For this review, take the finished solid that the model builds, in its own axes (mm). Face numbers are marked on the shaded views. A direction names the side the tool comes from. Coordinates: 2 decimals unless noted, no trailing zeros. Write each loop counter-clockwise with the first axis right and the second up, starting at its lowest first coordinate (ties: lowest second). Pieces come first, ordered by that corner, then holes.
1) We need section B-B on x = 80. Write out the cut boundary in (y, z), then the cut area to 3 significant figures.
2) Mouldability with a two-part tool opening along X and no side actions: class the marked faces 1 and 2 as pulls with the +X half, pulls with the -X half, needs draft (parallel to the pull), parting line crosses it, or undercut.
3) We need section D-D on z = 70.5. Write out the cut boundary in (x, y).
4) Insertion check: P1, Ø1.5, axis at x = 69.5, y = -6.5, coming from the -Z side; P2, Ø6, axis at x = 139.5, z = 55, coming from the -Y side; P3, Ø6, axis at y = -3.5, z = 91.5, coming from the +X side; P4, Ø24, axis at x = 79, z = 55.5, coming from the +Y side. Each pin has a flat end and moves straight along its axis. Give the tip position at first contact, or say it passes through.
5) For the marked faces 3, 4 and 5, list the 3-axis set-ups (+Z, -Z, +X, -X, +Y, -Y) from which the entire face can be reached by the end or side of a thin tool; tool diameter is ignored.
6) We need section C-C on z = 24.5. Write out the cut boundary in (x, y).
7) To check wall thickness, follow line 1 along Z through (x, y) = (140, 2.1); line 2 along X through (y, z) = (2.45, 55); line 3 along X through (y, z) = (-8.75, 55). State the ranges of each line that lie inside material, in increasing order.
8) We need section A-A on y = -4.25. Write out the cut boundary in (x, z), then the cut area to 3 significant figures.
from build123d import *

# Parameters (mm, degrees)
SKETCH1_W           = 160
SKETCH1_H           = 110
BOSS_EXTRUDE1_DEPTH = 3
SKETCH2_R           = 47.5
BOSS_EXTRUDE3_DEPTH = 10
FILLET1_R           = 7
FILLET2_R           = 7
FILLET3_R           = 7
FILLET4_R           = 7
CUT_EXTRUDE3_DEPTH  = 12
SKETCH8_R           = 25
CUT_EXTRUDE4_DEPTH  = 12
SKETCH9_R           = 22.5
CUT_EXTRUDE5_DEPTH  = 15
SKETCH11_R          = 2.25
CUT_EXTRUDE7_DEPTH  = 9
SKETCH12_R          = 6
BOSS_EXTRUDE4_DEPTH = 2
CUT_EXTRUDE8_DEPTH  = 10
SKETCH10_R          = 25
CUT_EXTRUDE9_DEPTH  = 10


with BuildPart() as part:
    # Sketch1 → Boss-Extrude1 (new body)
    with BuildSketch(Plane(origin=(0, 0, 0), x_dir=(1, 0, 0), z_dir=(0, 1, 0))):
        with Locations((80, -55)):
            Rectangle(SKETCH1_W, SKETCH1_H)
    extrude(amount=BOSS_EXTRUDE1_DEPTH)

    # Sketch2 → Boss-Extrude3 (add)
    with BuildSketch(Plane.XZ):
        with Locations(Location((80, 55, 0), (0, 0, 270))):
            Circle(SKETCH2_R)
    extrude(amount=BOSS_EXTRUDE3_DEPTH)

    # Fillet1
    fillet1_edges = [part.edges().sort_by_distance(p)[0] for p in [
        (160, 1.5, 110),
    ]]
    fillet(fillet1_edges, radius=FILLET1_R)

    # Fillet2
    fillet2_edges = [part.edges().sort_by_distance(p)[0] for p in [
        (160, 1.5, 0),
    ]]
    fillet(fillet2_edges, radius=FILLET2_R)

    # Fillet3
    fillet3_edges = [part.edges().sort_by_distance(p)[0] for p in [
        (0, 1.5, 0),
    ]]
    fillet(fillet3_edges, radius=FILLET3_R)

    # Fillet4
    fillet4_edges = [part.edges().sort_by_distance(p)[0] for p in [
        (0, 1.5, 110),
    ]]
    fillet(fillet4_edges, radius=FILLET4_R)

    # Sketch3 → Cut-Extrude3 (cut)
    with BuildSketch(Plane(origin=(0, 3, 0), x_dir=(1, 0, 0), z_dir=(0, 1, 0))):
        with BuildLine():
            ThreePointArc((45.034735386, -74.427564708), (51.715728753, -83.284271247), (60.572435292, -89.965264614))
            ThreePointArc((60.572435292, -89.965264614), (48.180194847, -86.819805153), (45.034735386, -74.427564708))
        make_face()
        with BuildLine():
            ThreePointArc((60.572435292, -20.034735386), (48.180194847, -23.180194847), (45.034735386, -35.572435292))
            ThreePointArc((45.034735386, -35.572435292), (51.715728753, -26.715728753), (60.572435292, -20.034735386))
        make_face()
        with BuildLine():
            ThreePointArc((114.965264614, -35.572435292), (111.819805153, -23.180194847), (99.427564708, -20.034735386))
            ThreePointArc((99.427564708, -20.034735386), (108.284271247, -26.715728753), (114.965264614, -35.572435292))
        make_face()
        with BuildLine():
            ThreePointArc((99.427564708, -89.965264614), (111.819805153, -86.819805153), (114.965264614, -74.427564708))
            ThreePointArc((114.965264614, -74.427564708), (108.284271247, -83.284271247), (99.427564708, -89.965264614))
        make_face()
    extrude(amount=-CUT_EXTRUDE3_DEPTH, mode=Mode.SUBTRACT)

    # Sketch8 → Cut-Extrude4 (cut)
    with BuildSketch(Plane(origin=(0, 3, 0), x_dir=(1, 0, 0), z_dir=(0, 1, 0))):
        with BuildLine():
            ThreePointArc((40.144230769, -58.393767674), (120, -55), (40.144230769, -51.606232326))
            ThreePointArc((40.144230769, -51.606232326), (40.30249314, -52.236544193), (40.814732143, -52.636483227))
            ThreePointArc((40.814732143, -52.636483227), (42.5, -55), (40.814732143, -57.363516773))
            ThreePointArc((40.814732143, -57.363516773), (40.30249314, -57.763455807), (40.144230769, -58.393767674))
        make_face()
        with Locations(Location((80, -55, 0), (0, 0, 270))):
            Circle(SKETCH8_R, mode=Mode.SUBTRACT)
    extrude(amount=-CUT_EXTRUDE4_DEPTH, mode=Mode.SUBTRACT)

    # Sketch9 → Cut-Extrude5 (cut)
    with BuildSketch(Plane(origin=(0, 3, 0), x_dir=(1, 0, 0), z_dir=(0, 1, 0))):
        with Locations(Location((80, -55, 0), (0, 0, 270))):
            Circle(SKETCH9_R)
    extrude(amount=-CUT_EXTRUDE5_DEPTH, mode=Mode.SUBTRACT)

    # Sketch11 → Cut-Extrude7 (cut)
    with BuildSketch(Plane(origin=(0, 3, 0), x_dir=(1, 0, 0), z_dir=(0, 1, 0))):
        with Locations(Location((20, -55, 0), (0, 0, 270))):
            Circle(SKETCH11_R)
        with Locations(Location((140, -55, 0), (0, 0, 270))):
            Circle(SKETCH11_R)
    extrude(amount=-CUT_EXTRUDE7_DEPTH, mode=Mode.SUBTRACT)

    # Sketch12 → Boss-Extrude4 (add)
    # profile 1 of 2: a face of its own
    with BuildSketch(Plane.XZ):
        with Locations(Location((20, 55, 0), (0, 0, 270))):
            Circle(SKETCH12_R)
        with BuildLine():
            Line((23.75277675, 55.5), (22.309401077, 58))
            ThreePointArc((22.309401077, 58), (21.943375673, 58.366025404), (21.443375673, 58.5))
            Line((21.443375673, 58.5), (18.556624327, 58.5))
            ThreePointArc((18.556624327, 58.5), (18.056624327, 58.366025404), (17.690598923, 58))
            Line((17.690598923, 58), (16.24722325, 55.5))
            ThreePointArc((16.24722325, 55.5), (16.113248654, 55), (16.24722325, 54.5))
            Line((16.24722325, 54.5), (17.690598923, 52))
            ThreePointArc((17.690598923, 52), (18.056624327, 51.633974596), (18.556624327, 51.5))
            Line((18.556624327, 51.5), (21.443375673, 51.5))
            ThreePointArc((21.443375673, 51.5), (21.943375673, 51.633974596), (22.309401077, 52))
            Line((22.309401077, 52), (23.75277675, 54.5))
            ThreePointArc((23.75277675, 54.5), (23.886751346, 55), (23.75277675, 55.5))
        make_face(mode=Mode.SUBTRACT)
    # profile 2 of 2: a face of its own
    with BuildSketch(Plane.XZ):
        with Locations(Location((140, 55, 0), (0, 0, 90))):
            Circle(SKETCH12_R)
        with BuildLine():
            Line((137.690598923, 52), (136.24722325, 54.5))
            ThreePointArc((136.24722325, 54.5), (136.113248654, 55), (136.24722325, 55.5))
            Line((136.24722325, 55.5), (137.690598923, 58))
            ThreePointArc((137.690598923, 58), (138.056624327, 58.366025404), (138.556624327, 58.5))
            Line((138.556624327, 58.5), (141.443375673, 58.5))
            ThreePointArc((141.443375673, 58.5), (141.943375673, 58.366025404), (142.309401077, 58))
            Line((142.309401077, 58), (143.75277675, 55.5))
            ThreePointArc((143.75277675, 55.5), (143.886751346, 55), (143.75277675, 54.5))
            Line((143.75277675, 54.5), (142.309401077, 52))
            ThreePointArc((142.309401077, 52), (141.943375673, 51.633974596), (141.443375673, 51.5))
            Line((141.443375673, 51.5), (138.556624327, 51.5))
            ThreePointArc((138.556624327, 51.5), (138.056624327, 51.633974596), (137.690598923, 52))
        make_face(mode=Mode.SUBTRACT)
    extrude(amount=BOSS_EXTRUDE4_DEPTH)

    # Sketch13 → Cut-Extrude8 (cut)
    with BuildSketch(Plane(origin=(0, 3, 0), x_dir=(1, 0, 0), z_dir=(0, 1, 0))):
        with BuildLine():
            Line((10, -13), (10, -27))
            ThreePointArc((10, -27), (10.878679656, -29.121320344), (13, -30))
            Line((13, -30), (28.757359313, -30))
            ThreePointArc((28.757359313, -30), (29.90540961, -29.771638598), (30.878679656, -29.121320344))
            Line((30.878679656, -29.121320344), (44.878679656, -15.121320344))
            ThreePointArc((44.878679656, -15.121320344), (45.52899791, -11.851949703), (42.757359313, -10))
            Line((42.757359313, -10), (13, -10))
            ThreePointArc((13, -10), (10.878679656, -10.878679656), (10, -13))
        make_face()
        with BuildLine():
            Line((129.121320344, -29.121320344), (115.121320344, -15.121320344))
            ThreePointArc((115.121320344, -15.121320344), (114.47100209, -11.851949703), (117.242640687, -10))
            Line((117.242640687, -10), (147, -10))
            ThreePointArc((147, -10), (149.121320344, -10.878679656), (150, -13))
            Line((150, -13), (150, -27))
            ThreePointArc((150, -27), (149.121320344, -29.121320344), (147, -30))
            Line((147, -30), (131.242640687, -30))
            ThreePointArc((131.242640687, -30), (130.09459039, -29.771638598), (129.121320344, -29.121320344))
        make_face()
        with BuildLine():
            Line((150, -97), (150, -83))
            ThreePointArc((150, -83), (149.121320344, -80.878679656), (147, -80))
            Line((147, -80), (131.242640687, -80))
            ThreePointArc((131.242640687, -80), (130.09459039, -80.228361402), (129.121320344, -80.878679656))
            Line((129.121320344, -80.878679656), (115.121320344, -94.878679656))
            ThreePointArc((115.121320344, -94.878679656), (114.47100209, -98.148050297), (117.242640687, -100))
            Line((117.242640687, -100), (147, -100))
            ThreePointArc((147, -100), (149.121320344, -99.121320344), (150, -97))
        make_face()
        with BuildLine():
            Line((30.878679656, -80.878679656), (44.878679656, -94.878679656))
            ThreePointArc((44.878679656, -94.878679656), (45.52899791, -98.148050297), (42.757359313, -100))
            Line((42.757359313, -100), (13, -100))
            ThreePointArc((13, -100), (10.878679656, -99.121320344), (10, -97))
            Line((10, -97), (10, -83))
            ThreePointArc((10, -83), (10.878679656, -80.878679656), (13, -80))
            Line((13, -80), (28.757359313, -80))
            ThreePointArc((28.757359313, -80), (29.90540961, -80.228361402), (30.878679656, -80.878679656))
        make_face()
    extrude(amount=-CUT_EXTRUDE8_DEPTH, mode=Mode.SUBTRACT)

    # Sketch10 → Cut-Extrude9 (cut)
    with BuildSketch(Plane(origin=(0, 3, 0), x_dir=(1, 0, 0), z_dir=(0, 1, 0))):
        with Locations(Location((80, -55, 0), (0, 0, 270))):
            Circle(SKETCH10_R)
    extrude(amount=-CUT_EXTRUDE9_DEPTH, mode=Mode.SUBTRACT)


solid = part.part
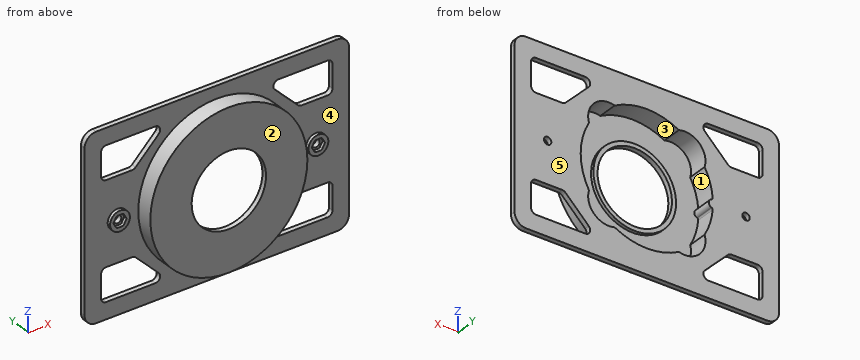
Result:
1. outline: (-10, 7.5) - (0, 7.5) - (0, 0) - (3, 0) - (3, 15) - (-9, 15) - (-9, 30) - (-7, 30) - (-7, 32.5) - (-10, 32.5) - close; (-10, 77.5) - (-7, 77.5) - (-7, 80) - (-9, 80) - (-9, 95) - (3, 95) - (3, 110) - (0, 110) - (0, 102.5) - (-10, 102.5) - close
1. area: 285 mm2
2. face 1: undercut
2. face 2: needs draft
3. outline: (0, 0) - (35.1, 0) - (35.1, -10) - (63.69, -10) - (63.69, -7) - (60.38, -7) - (60.38, -9) - (43.13, -9) - (43.13, 3) - (0, 3) - close; (96.31, -10) - (124.9, -10) - (124.9, 0) - (160, 0) - (160, 3) - (116.87, 3) - (116.87, -9) - (99.62, -9) - (99.62, -7) - (96.31, -7) - close
4. P1: stops at z = 8.51
4. P2: stops at y = 0
4. P3: stops at x = 113.67
4. P4: passes through
5. face 3: +Y
5. face 4: -Y
5. face 5: +Z, -Z, +X, -X, +Y
6. outline: (0, 0) - (10, 0) - (10, 3) - (0, 3) - close; (35.5, 0) - (43.59, 0) - (43.59, -10) - (116.41, -10) - (116.41, 0) - (124.5, 0) - (124.5, 3) - (112.97, 3) - (112.97, -9) - (47.03, -9) - (47.03, 3) - (35.5, 3) - close; (150, 0) - (160, 0) - (160, 3) - (150, 3) - close
7. line 1: z = 0 to 10, 30 to 52.75, 57.25 to 80, 100 to 110
7. line 2: x = 0 to 17.75, 22.25 to 42.5, 120 to 137.75, 142.25 to 160
7. line 3: x = 32.5 to 42.5, 55 to 57.5, 102.5 to 105, 120 to 127.5
8. outline: circle Ø95 at (80, 55); hole (40.14, 51.61) arc R40 ccw to (45.03, 35.57) arc R12.5 ccw to (60.57, 20.03) arc R40 ccw to (99.43, 20.03) arc R12.5 ccw to (114.97, 35.57) arc R40 ccw to (114.97, 74.43) arc R12.5 ccw to (99.43, 89.97) arc R40 ccw to (60.57, 89.97) arc R12.5 ccw to (45.03, 74.43) arc R40 ccw to (40.14, 58.39) arc R1 ccw to (40.81, 57.36) arc R2.5 cw to (40.81, 52.64) arc R1 ccw to start
8. area: 1,750 mm2
